Autodesk Inventor part; units mm, degrees
ref_plane "YZ Plane" through (0, 0, 0) normal (1, 0, 0) x (0, 1, 0)
ref_plane "XZ Plane" through (0, 0, 0) normal (0, 1, 0) x (-1, 0, 0)
ref_plane "XY Plane" through (0, 0, 0) normal (0, 0, 1) x (1, 0, 0)
sketch "スケッチ1" plane through (0, 0, 0) normal (0, 1, 0) x (-1, 0, 0)
  line L0 (-277.5, 280) -> (277.5, 280)
  line L1 (277.5, 280) -> (277.5, -280)
  line L2 (277.5, -280) -> (-277.5, -280)
  line L3 (-277.5, -280) -> (-277.5, 280)
  line L4 (-277.5, 280) -> (277.5, -280) construction
  line L5 (277.5, 280) -> (-277.5, -280) construction
  point P0 (0, 0)
  dimension "d0" = 555
  dimension "d1" = 560
extrude "押し出し1" add sketch "スケッチ1" along normal mid plane 5
sketch "スケッチ3" plane through (0, -2.5, 0) normal (0, -1, 0) x (1, 0, 0)
  circle A0 centre (-62.5, 115) radius 2.5
  line L0 (277.5, -280) -> (277.5, 280)
  line L1 (-277.5, -280) -> (277.5, -280)
  circle A1 centre (-162.5, 190) radius 2.5
  circle A2 centre (257.5, 40) radius 2.5
  point P0 (0, 0)
  dimension "d10" = 5
  dimension "d15" = 5
  dimension "d16" = 320
  dimension "d17" = 20
  dimension "d18" = 5
  dimension "d24" = 75
  dimension "d25" = 320
  dimension "d26" = 420
  dimension "d27" = 150
extrude "押し出し4" cut sketch "スケッチ3" against normal through all
sketch "スケッチ5" plane through (0, -2.5, 0) normal (0, -1, 0) x (1, 0, 0)
  line L0 (277.5, 250) -> (-277.5, 250)
  line L1 (-250, 280) -> (-250, -280) construction
  line L2 (-277.5, -250) -> (277.5, -250)
  line L3 (250, -280) -> (250, 280) construction
  line L4 (-277.5, 280) -> (277.5, 280)
  line L5 (-150, 280) -> (277.5, 120)
  line L6 (277.5, 280) -> (277.5, -280)
  line L7 (-277.5, -280) -> (-277.5, 280)
  line L8 (-277.5, 120) -> (-150.482941, -100)
  line L9 (-150.482941, -100) -> (277.5, -100)
  line L10 (277.5, -280) -> (277.5, 280)
  point P0 (0, 0)
  dimension "d32" = 100
  dimension "d33" = 130
  dimension "d34" = 350
  dimension "d35" = 60
  dimension "d46" = 220
sketch "スケッチ5 outline for 押し出し5" plane through (0, -2.5, 0) normal (0, -1, 0) x (1, 0, 0)
  line L0 (277.5, 120) -> (277.5, 280)
  line L1 (-150, 280) -> (277.5, 120)
  line L2 (277.5, 280) -> (-150, 280)
  line L3 (-277.5, 120) -> (-277.5, -280)
  line L4 (-150.482941, -100) -> (-277.5, 120)
  line L5 (277.5, -100) -> (-150.482941, -100)
  line L6 (277.5, -280) -> (277.5, -100)
  line L7 (-277.5, -280) -> (277.5, -280)
extrude "押し出し5" cut sketch "スケッチ5 outline for 押し出し5" against normal through all
chamfer "面取り2" distance 170 distance2 100 1 edges at (-150.4829, 0, -100) measured on face at (134.839, -0.8333, -100)
properties part number "endplate"
Part model, mm, in its own coordinate system. Give positions to 0.01 mm unless a question says otherwise; leave off trailing zeros. Write each loop counter-clockwise with the first axis right and the second up, starting at its lowest first coordinate (ties: lowest second). Pieces come first, ordered by that corner, then holes.
1) Cut at C-C on z = 151.5. Write the cut outline in (x, y), then the cut area to 3 significant figures.
Resolved:
outline: (-277.5, -2.5) - (193.34, -2.5) - (193.34, 2.5) - (-277.5, 2.5) - close
area: 2,350 mm2
2) Probe L1, parallel to Z at x = -162.5, y = 1.2; L2, parallel to Z at x = -62.5, y = 0.4; L3, parallel to Z at x = -50, y = -0.05. List the from-to ranges inside material, lowest first.
Resolved:
L1: z = -28.35 to 187.5, 192.5 to 280
L2: z = -67.71 to 112.5, 117.5 to 247.25
L3: z = -72.63 to 242.57
3) Pin check, flat tip, straight feed: pin 1 (1 mm diameter, centred on x = 149.5, y = 1, fed in from +Z). Stop position of the tip, or through.
Resolved:
pin 1: stops at z = 168.09
4) Cut at B-B on x = -35.5. Write the cut outline in (y, z), then the cut area to 3 significant figures.
Resolved:
outline: (-2.5, -78.34) - (2.5, -78.34) - (2.5, 237.15) - (-2.5, 237.15) - close
area: 1,580 mm2
5) Cut at A-A on y = -0.25. Write the cut outline in (x, z), then the cut area to 3 significant figures.
Resolved:
outline: (-277.5, 120) - (-200.48, -13.4) - (19.52, -100) - (277.5, -100) - (277.5, 120) - (-150, 280) - (-277.5, 280) - close; hole circle Ø5 at (-162.5, 190); hole circle Ø5 at (-62.5, 115); hole circle Ø5 at (257.5, 40)
area: 155,000 mm2
